```python
from build123d import *

# Parameters (mm, degrees)
IZIM1_R                     = 1.5
IZIM1_R_2                   = 5
Y_KSEKLIK_EKSTR_ZYON1_DEPTH = 2
CHAMFER_1_SIZE              = 1


with BuildPart() as part:
    # Çizim1 → Yükseklik-Ekstrüzyon1 (new body)
    with BuildSketch(Plane.XY):
        with BuildLine():
            Line((10, 4), (16.5, 4))
            ThreePointArc((16.5, 4), (20.500000347, 3.47e-07), (16.500000694, -4))
            Line((16.500000694, -4), (10.000000694, -4))
            ThreePointArc((10.000000694, -4), (5.757359762, -5.757359558), (4.000000694, -10.000000694))
            Line((4.000000694, -10.000000694), (4.000000694, -16.500000694))
            ThreePointArc((4.000000694, -16.500000694), (6.94e-07, -20.500000694), (-3.999999306, -16.500000694))
            Line((-3.999999306, -16.500000694), (-3.999999306, -10.000000694))
            ThreePointArc((-3.999999306, -10.000000694), (-5.757358864, -5.757359762), (-10, -4.000000694))
            Line((-10, -4.000000694), (-16.5, -4.000000694))
            ThreePointArc((-16.5, -4.000000694), (-20.5, -6.94e-07), (-16.5, 3.999999306))
            Line((-16.5, 3.999999306), (-10, 3.999999306))
            ThreePointArc((-10, 3.999999306), (-5.757359067, 5.757358864), (-4, 10))
            Line((-4, 10), (-4, 16.5))
            ThreePointArc((-4, 16.5), (0, 20.5), (4, 16.5))
            Line((4, 16.5), (4, 10))
            ThreePointArc((4, 10), (5.757359313, 5.757359313), (10, 4))
        make_face()
        with Locations((0, 8)):
            Circle(IZIM1_R, mode=Mode.SUBTRACT)
        with Locations((16.500000347, 0)):
            Circle(IZIM1_R, mode=Mode.SUBTRACT)
        with Locations((9.5, -6.94e-07)):
            Circle(IZIM1_R, mode=Mode.SUBTRACT)
        with Locations((0, 16.5)):
            Circle(IZIM1_R, mode=Mode.SUBTRACT)
        with Locations((6.94e-07, -16.500000694)):
            Circle(IZIM1_R, mode=Mode.SUBTRACT)
        with Locations((6.94e-07, -8.000000694)):
            Circle(IZIM1_R, mode=Mode.SUBTRACT)
        Circle(IZIM1_R_2, mode=Mode.SUBTRACT)
        with Locations((-16.5, -6.94e-07)):
            Circle(IZIM1_R, mode=Mode.SUBTRACT)
        with Locations((-9.5, -6.94e-07)):
            Circle(IZIM1_R, mode=Mode.SUBTRACT)
    extrude(amount=Y_KSEKLIK_EKSTR_ZYON1_DEPTH)

    # Фаска1
    chamfer_1_edges = [part.edges().sort_by_distance(p)[0] for p in [
        (-1.5, 8, 0),
        (8, -6.94e-07, 0),
        (-1.499999306, -8.000000694, 0),
        (-11, -6.94e-07, 0),
    ]]
    chamfer(chamfer_1_edges, length=CHAMFER_1_SIZE)


solid = part.part
```
Geometry: final body of the model. Coordinates: model frame, mm. A direction names the side the tool comes from. Give positions to 0.01 mm unless a question says otherwise; leave off trailing zeros. Order: outer loops, then holes, each group sorted by start corner. A loop starts at its lowest first (then second) coordinate and runs counter-clockwise, first axis right, second up. Notation, with made-up numbers: (32.25, 69.5) -> (68.25, 69.5) arc R30 ccw to (68.25, 98.5) -> close; hole circle Ø2 at (12.25, 53). An arc over 180 degrees is marked (long way). Write each question's results on one line, items separated by ' | '. Start each with the question number.
1) First-contact query: pin 1 (1 mm diameter, centred on x = 14.5, z = 1, fed in from +Y); pin 2 (0.6 mm diameter, centred on y = 15, z = 1, fed in from +X). Flat tips, straight axial feed; report the tip coordinate or a pass-through.
2) Section B-B (x = 3.5). Return loops of the section in (y, z).
3) Line query: line 1 (Y direction, x = 0, z = 1.25); line 2 (Y direction, x = 0, z = 0.5); line 3 (X direction, y = -16.5, z = 1.2). Output: solid intervals per line, ascending. Write a range as from..to.
4) Section D-D (x = -9.5). Return loops of the section in (y, z), then the cut area to 3 significant figures.
5) Section A-A (z = 0.4). Count the separate pieces of the cut face and the enclosed holes in it, then the cut area to 3 significant figures.
6) Section C-C (y = 4.5). Return loops of the section in (x, z).
7) Draft query along Z for faces 6 (the cylindrical face through (-18, 0, 1)), 7 (the flat face through (3.1, -4.5, 2)). Return one class per face: pulls with the +Z half, pulls with the -Z half, needs draft (parallel to the pull), parting line crosses it, or undercut.
8) Set-up query: faces 1 (the flat face through (13, -4, 1)), 2 (the cylindrical face through (-1.08, -4.88, 0.99)), 3 (the flat face through (-4, 13, 1)), 4 (the flat face through (-13, -4, 1)), 5 (the cylindrical face through (-0.1, 20.5, 1)). Return all of +Z, -Z, +X, -X, +Y, -Y with unobstructed straight access to the full face (end or side cutting, diameter ignored); none if empty.
Calculated:
1) pin 1: y = 4 | pin 2: x = 4
2) outline: (-18.44, 0) -> (-3.57, 0) -> (-3.57, 2) -> (-18.44, 2) -> close; (3.57, 0) -> (18.44, 0) -> (18.44, 2) -> (3.57, 2) -> close
3) line 1: -20.5..-18, -15..-9.5, -6.5..-5, 5..6.5, 9.5..15, 18..20.5 | line 2: -20.5..-18, -15..-10, -6..-5, 5..6, 10..15, 18..20.5 | line 3: -4..-1.5, 1.5..4
4) outline: (-4.02, 0) -> (-2.5, 0) -> (-1.5, 1) -> (-1.5, 2) -> (-4.02, 2) -> close; (1.5, 1) -> (2.5, 0) -> (4.02, 0) -> (4.02, 2) -> (1.5, 2) -> close | area: 9.08 mm2
5) separate pieces: 1 | enclosed holes: 9 | area: 433 mm2
6) outline: (-7.6, 0) -> (-2.18, 0) -> (-2.18, 2) -> (-7.6, 2) -> close; (2.18, 0) -> (7.6, 0) -> (7.6, 2) -> (2.18, 2) -> close
7) face 6: needs draft | face 7: pulls with the +Z half
8) face 1: +Z, -Z, +X, -Y | face 2: +Z, -Z | face 3: +Z, -Z, -X, +Y | face 4: +Z, -Z, -X, -Y | face 5: +Z, -Z, +Y
